Source: CAD feature listing. Evaluate the final solid. Frame: model axes, mm. A direction names the side the tool comes from. Give positions to 0.01 mm unless a question says otherwise; leave off trailing zeros. Order: outer loops, then holes, each group sorted by start corner. A loop starts at its lowest first (then second) coordinate and runs counter-clockwise, first axis right, second up.
from build123d import *

# Parameters (mm, degrees)
FILLET_2_R = 0.5


with BuildPart() as part:
    # 草图1 → 旋转1 (revolve)
    with BuildSketch(Plane.XY, mode=Mode.PRIVATE) as revolve_1_sk:
        Polygon((2, 7), (7.5, 7), (6.5, 0), (3.5, 0), (3.5, 3.27), (2, 3.27), align=None)
    revolve(revolve_1_sk.sketch.rotate(Axis((0, 0, 0), (0, 1, 0)), 90), axis=Axis((0, 0, 0), (0, 1, 0)))

    # 圆角2
    fillet_2_edges = [part.edges().sort_by_distance(p)[0] for p in [
        (0, 0, 3.5),
        (0, 0, 6.5),
    ]]
    fillet(fillet_2_edges, radius=FILLET_2_R)


solid = part.part
1) Ray query, L1, parallel to X at y = 2.75, z = -0.5; L2, parallel to X at y = 3, z = 2.5; L3, parallel to Z at x = -1.25, y = 2.5. Return the intervals inside material, ascending.
Checks:
L1: x = -6.87 to -3.46, 3.46 to 6.87
L2: x = -6.46 to -2.45, 2.45 to 6.46
L3: z = -6.74 to -3.27, 3.27 to 6.74
2) Section query D-D on y = 5.75. Output: boundary loops of the cut face in (x, z).
Checks:
outline: circle Ø14.64 at (0, 0); hole circle Ø4 at (0, 0)
3) Section query B-B on z = 0. Output: boundary loops of the cut face in (x, y).
Checks:
outline: (-7.5, 7) - (-6.56, 0.43) arc R0.5 ccw to (-6.07, 0) - (-4, 0) arc R0.5 ccw to (-3.5, 0.5) - (-3.5, 3.27) - (-2, 3.27) - (-2, 7) - close; (2, 3.27) - (3.5, 3.27) - (3.5, 0.5) arc R0.5 ccw to (4, 0) - (6.07, 0) arc R0.5 ccw to (6.56, 0.43) - (7.5, 7) - (2, 7) - close
4) Section query A-A on x = 0. Output: boundary loops of the cut face in (y, z), and give its area (3 significant figures).
Checks:
outline: (0, -6.07) arc R0.5 ccw to (0.43, -6.56) - (7, -7.5) - (7, -2) - (3.27, -2) - (3.27, -3.5) - (0.5, -3.5) arc R0.5 ccw to (0, -4) - close; (0, 4) arc R0.5 ccw to (0.5, 3.5) - (3.27, 3.5) - (3.27, 2) - (7, 2) - (7, 7.5) - (0.43, 6.56) arc R0.5 ccw to (0, 6.07) - close
area: 60.0 mm2
5) First-contact query: pin 1 Ø3 at (x, y) = (4, 4) entering from +Z; pin 2 Ø5.5 at (x, z) = (0, 0.5) entering from -Y; pin 3 Ø4 at (x, y) = (0, 1.5) entering from +Z. Flat tips, straight axial feed; report the tip coordinate or a pass-through.
Checks:
pin 1: stops at z = 6.66
pin 2: stops at y = 3.27
pin 3: stops at z = 7
6) Pull-direction query (X, two-part tool) for faces 1 (the face through (3.105, 1.904, -1.615)), 2 (the face through (2, 7, 2)), 3 (the face through (-2.08, 2.94, -6.6)), 4 (the face through (2, 5, 0)); classes: +X half, -X half, draft (parallel to the pull), parting line (faces both ways), or undercut.
Checks:
face 1: undercut
face 2: draft
face 3: parting line
face 4: undercut
7) Section query C-C on y = 3.75. Output: boundary loops of the cut face in (x, z).
Checks:
outline: circle Ø14.07 at (0, 0); hole circle Ø4 at (0, 0)
8) Reachability of faces 5 (the face through (2, 3.27, -2)), 6 (the face through (4, 0, -1.3)) from +Z, -Z, +X, -X, +Y, -Y: full face, straight path, thin tool, end or side. Return the list, or none.
Checks:
face 5: -Y
face 6: +Z, -Z, +X, -X, -Y
